from build123d import *

# Parameters (mm, degrees)
BOSS_EXTRUDE1_DEPTH = 50.8
SKETCH2_R           = 19.939
BOSS_EXTRUDE2_DEPTH = 83.82
BOSS_EXTRUDE3_DEPTH = 171.704
BOSS_EXTRUDE4_DEPTH = 20.066
SKETCH5_R           = 3.81
CUT_EXTRUDE1_DEPTH  = 20.066
SKETCH6_R           = 9.906
CUT_EXTRUDE2_DEPTH  = 127


with BuildPart() as part:
    # Sketch1 → Boss-Extrude1 (new body)
    with BuildSketch(Plane(origin=(0, 0, 0), x_dir=(1, 0, 0), z_dir=(0, 1, 0))):
        with BuildLine():
            Line((-50.83623546, -27.655683544), (-45.75623546, -32.735683544))
            Line((-45.75623546, -32.735683544), (-14.00623546, -32.735683544))
            Line((-14.00623546, -32.735683544), (-8.92623546, -27.655683544))
            Line((-8.92623546, -27.655683544), (-8.92623546, 28.376716456))
            ThreePointArc((-8.92623546, 28.376716456), (-15.056373373, 43.176178544), (-29.85583546, 49.306316456))
            Line((-29.85583546, 49.306316456), (-29.90663546, 49.306316456))
            ThreePointArc((-29.90663546, 49.306316456), (-44.706097548, 43.176178544), (-50.83623546, 28.376716456))
            Line((-50.83623546, 28.376716456), (-50.83623546, -27.655683544))
        make_face()
    extrude(amount=BOSS_EXTRUDE1_DEPTH)

    # Sketch2 → Boss-Extrude2 (add)
    with BuildSketch(Plane(origin=(0, 50.8, 0), x_dir=(1, 0, 0), z_dir=(0, 1, 0))):
        with Locations((-29.88123546, 28.351316456)):
            Circle(SKETCH2_R)
    extrude(amount=BOSS_EXTRUDE2_DEPTH)

    # Sketch3 → Boss-Extrude3 (add)
    with BuildSketch(Plane(origin=(0, 50.8, 0), x_dir=(1, 0, 0), z_dir=(0, 1, 0))):
        with BuildLine():
            Line((-45.12123546, -31.707852889), (-14.64123546, -31.707852889))
            Line((-14.64123546, -31.707852889), (-14.64123546, -10.371852889))
            ThreePointArc((-14.64123546, -10.371852889), (-29.88123546, 4.868147111), (-45.12123546, -10.371852889))
            Line((-45.12123546, -10.371852889), (-45.12123546, -31.707852889))
        make_face()
    extrude(amount=BOSS_EXTRUDE3_DEPTH)

    # Sketch4 → Boss-Extrude4 (add)
    with BuildSketch(Plane(origin=(0, 0, 0), x_dir=(-1, 0, 0), z_dir=(0, -1, 0))):
        with BuildLine():
            Line((24.67423546, 0.157316456), (35.08823546, 0.157316456))
            ThreePointArc((35.08823546, 0.157316456), (37.782312297, -0.958606708), (38.89823546, -3.652683544))
            Line((38.89823546, -3.652683544), (38.89823546, -14.066683544))
            ThreePointArc((38.89823546, -14.066683544), (37.782312297, -16.76076038), (35.08823546, -17.876683544))
            Line((35.08823546, -17.876683544), (24.67423546, -17.876683544))
            ThreePointArc((24.67423546, -17.876683544), (21.980158624, -16.76076038), (20.86423546, -14.066683544))
            Line((20.86423546, -14.066683544), (20.86423546, -3.652683544))
            ThreePointArc((20.86423546, -3.652683544), (21.980158624, -0.958606708), (24.67423546, 0.157316456))
        make_face()
    extrude(amount=BOSS_EXTRUDE4_DEPTH)

    # Sketch5 → Cut-Extrude1 (cut)
    with BuildSketch(Plane.ZY.offset(38.89823546)):
        with Locations((8.859683544, -11.938)):
            Circle(SKETCH5_R)
    extrude(amount=-CUT_EXTRUDE1_DEPTH, mode=Mode.SUBTRACT)

    # Sketch6 → Cut-Extrude2 (cut)
    with BuildSketch(Plane(origin=(0, 222.504, 0), x_dir=(1, 0, 0), z_dir=(0, 1, 0))):
        with Locations((-29.88123546, -8.859683544)):
            Circle(SKETCH6_R)
    extrude(amount=-CUT_EXTRUDE2_DEPTH, mode=Mode.SUBTRACT)


solid = part.part
Read the model definition and answer for the solid it produces. Units are mm, in the model's axes. A direction names the side the tool comes from. Give positions to 0.01 mm unless a question says otherwise; leave off trailing zeros. Write each loop counter-clockwise with the first axis right and the second up, starting at its lowest first coordinate (ties: lowest second). Pieces come first, ordered by that corner, then holes. Notation, with made-up numbers: (43, 62) -> (80, 62) arc R34 ccw to (80, 98) -> close; hole circle Ø1 at (81.5, 41.5). An arc over 180 degrees is marked (long way). Answer as a JSON object with one key per item and string values. Group by question number.
1) A tool of negligible diameter and unlimited length cuts with its end or side. For faces 1 (the cylindrical face through (-29.546, 135.45, -4.864)), 2 (the flat face through (-38.898, -7.7, 8.8)), 3 (the flat face through (-30, -10, -0.157)), from which of +Z, -Z, +X, -X, +Y, -Y can it reach the whole face along a straight path? Write none if from no direction.
2) Find section A-A (y = 18.5). Write down the section's boundary in (x, z).
3) Each of these flat-tipped pins is pushed along its axis until it touches: P1, Ø16, axis at x = -29.88, z = 8.86, coming from the +Y side; P2, Ø1.5, axis at x = -14, y = 108, coming from the -Z side; P3, Ø4, axis at y = 89.5, z = 7.5, coming from the -X side; P4, Ø11.5, axis at y = -5.5, z = 6.5, coming from the -X side. Where does it stop, or does it pass through?
4) Find section D-D (y = 148.5). Write down the section's boundary in (x, z).
5) The mould has two halves that part along Z. Classify faces 4 (the cylindrical face through (-30.007, -11.77, 5.053)), 5 (the cylindrical face through (-20.433, 159.893, 5.884)), 6 (the flat face through (-11.5, 25.04, 30.23)), 7 (the flat face through (-30, 134.62, -29)): +Z half, -Z half, draft (parallel to the pull), parting line (faces both ways), or undercut.
6) Find section C-C (z = -11.5). Write down the section's boundary in (x, y), and give its area (3 significant figures).
7) Consider L1, parallel to Y at x = -34.5, z = 8.5; L2, parallel to Y at x = -12, z = -25; L3, parallel to Y at x = -14.5, z = 13.5. Determine where each line is inside the solid, lowest interval first. Write a range as from..to.
8) Find section B-B (y = 76). Write down the section's boundary in (x, z), and give its area (3 significant figures).
Values follow:
{
 "1": {"face 1": "+Y", "face 2": "+Z, -Z, -X, -Y", "face 3": "-Z, +X, -X, -Y"},
 "2": {"outline": "(-50.84, -28.38) arc R20.93 ccw to (-29.91, -49.31) -> (-29.86, -49.31) arc R20.93 ccw to (-8.93, -28.38) -> (-8.93, 27.66) -> (-14.01, 32.74) -> (-45.76, 32.74) -> (-50.84, 27.66) -> close"},
 "3": {"P1": "stops at y = 95.5", "P2": "stops at z = -41.34", "P3": "stops at x = -45.1", "P4": "stops at x = -50.84"},
 "4": {"outline": "(-45.12, 10.37) arc R15.24 ccw to (-14.64, 10.37) -> (-14.64, 31.71) -> (-45.12, 31.71) -> close; hole circle Ø19.81 at (-29.88, 8.86)"},
 "5": {"face 4": "undercut", "face 5": "undercut", "face 6": "+Z half", "face 7": "draft"},
 "6": {"outline": "(-50.84, 0) -> (-8.93, 0) -> (-8.93, 50.8) -> (-19.22, 50.8) -> (-19.22, 134.62) -> (-40.54, 134.62) -> (-40.54, 50.8) -> (-50.84, 50.8) -> close", "area": "3,920 mm2"},
 "7": {"L1": "y = -20.07..-15.73, -8.15..95.5", "L2": "y = 0..134.62", "L3": "y = 0..50.8"},
 "8": {"outline": "circle Ø39.88 at (-29.88, -28.35); (-45.12, 10.37) arc R15.24 ccw to (-14.64, 10.37) -> (-14.64, 31.71) -> (-45.12, 31.71) -> close", "area": "2,260 mm2"}
}
